Design review of the part built by this model. Coordinates are the model's own, in mm. A direction names the side the tool comes from. Coordinates: 2 decimals unless noted, no trailing zeros. Write each loop counter-clockwise with the first axis right and the second up, starting at its lowest first coordinate (ties: lowest second). Pieces come first, ordered by that corner, then holes. Notation, with made-up numbers: M 75,-33 L 131,-33 A16 ccw 131,-12 Z; hole C 9,87 d7. An arc over 180 degrees is marked long. Return JSON: item names as keys, results as strings. Group by question number.
```python
from build123d import *

# Parameters (mm, degrees)
CROQUIS1_W                = 110
CROQUIS1_H                = 60
SALIENTE_EXTRUIR1_DEPTH   = 5
SALIENTE_EXTRUIR2_DEPTH   = 45
CROQUIS4_W                = 15
CROQUIS4_H                = 15
SALIENTE_EXTRUIR3_DEPTH   = 15
CROQUIS5_W                = 15
CROQUIS5_H                = 15
CORTAR_EXTRUIR1_DEPTH     = 5
TALADRO_ROSCADO_M41_D     = 3.3
TALADRO_ROSCADO_M41_DEPTH = 14.008579979
TALADRO_ROSCADO_M41_TIP   = 0.991420021
CROQUIS11_W               = 5
CROQUIS11_H               = 4
SALIENTE_EXTRUIR4_DEPTH   = 3
CROQUIS12_W               = 40
CROQUIS12_H               = 4
SALIENTE_EXTRUIR5_DEPTH   = 2


with BuildPart() as part:
    # Croquis1 → Saliente-Extruir1 (new body)
    with BuildSketch(Plane(origin=(0, 0, 0), x_dir=(1, 0, 0), z_dir=(0, 1, 0))):
        with Locations((55, 30)):
            Rectangle(CROQUIS1_W, CROQUIS1_H)
    extrude(amount=SALIENTE_EXTRUIR1_DEPTH)

    # Croquis2 → Saliente-Extruir2 (add)
    with BuildSketch(Plane(origin=(0, 5, 0), x_dir=(1, 0, 0), z_dir=(0, 1, 0))):
        Polygon((0, 0), (10, 0), (10, 15), (5, 15), (5, 45), (10, 45), (10, 60), (0, 60), align=None)
    extrude(amount=SALIENTE_EXTRUIR2_DEPTH)

    # Croquis4 → Saliente-Extruir3 (add)
    with BuildSketch(Plane(origin=(0, 5, 0), x_dir=(1, 0, 0), z_dir=(0, 1, 0))):
        with Locations((102.5, 52.5)):
            Rectangle(CROQUIS4_W, CROQUIS4_H)
        with Locations((102.5, 7.5)):
            Rectangle(CROQUIS4_W, CROQUIS4_H)
    extrude(amount=SALIENTE_EXTRUIR3_DEPTH)

    # Croquis5 → Cortar-Extruir1 (cut)
    with BuildSketch(Plane(origin=(110, 0, 0), x_dir=(0, 0, -1), z_dir=(1, 0, 0))):
        with Locations((7.5, 12.5)):
            Rectangle(CROQUIS5_W, CROQUIS5_H)
        with Locations((52.5, 12.5)):
            Rectangle(CROQUIS5_W, CROQUIS5_H)
    extrude(amount=-CORTAR_EXTRUIR1_DEPTH, mode=Mode.SUBTRACT)

    # Taladro roscado M41
    with Locations(Plane(origin=(105, 0, 0), x_dir=(0, 0, -1), z_dir=(1, 0, 0))):
        with Locations((7.5, 12.5), (52.5, 12.5)):
            Hole(TALADRO_ROSCADO_M41_D / 2, depth=TALADRO_ROSCADO_M41_DEPTH)
            with Locations((0, 0, -(TALADRO_ROSCADO_M41_DEPTH + TALADRO_ROSCADO_M41_TIP / 2))):  # 118° drill point
                Cone(0, TALADRO_ROSCADO_M41_D / 2, TALADRO_ROSCADO_M41_TIP, mode=Mode.SUBTRACT)

    # Croquis11 → Saliente-Extruir4 (add)
    with BuildSketch(Plane.ZY):
        with Locations((-47.5, 32)):
            Rectangle(CROQUIS11_W, CROQUIS11_H)
        with Locations((-12.5, 32)):
            Rectangle(CROQUIS11_W, CROQUIS11_H)
    extrude(amount=SALIENTE_EXTRUIR4_DEPTH)

    # Croquis12 → Saliente-Extruir5 (add)
    with BuildSketch(Plane.ZY.offset(3)):
        with Locations((-30, 32)):
            Rectangle(CROQUIS12_W, CROQUIS12_H)
    extrude(amount=SALIENTE_EXTRUIR5_DEPTH)


solid = part.part
```
Item 1: Add section C-C (x = 7.5). Write out the cut boundary in (y, z), plus the area to 3 significant figures.
Item 2: The part is to be moulded in two halves that separate along X. For faces 4 (the flat face through (-1, 32, -45)), 5 (the flat face through (105, 14.3, -7.4)), 6 (the flat face through (54, 0, -30)), 7 (the flat face through (10, 27, -52)), say which applies: pulls with the +X half, pulls with the -X half, needs draft (parallel to the pull), parting line crosses it, or undercut.
Item 3: Machinability: for faces 1 (the flat face through (-2, 32, -10)), 2 (the flat face through (-3, 32, -30)), 3 (the flat face through (8, 27, -15)), which of the approach directions +Z, -Z, +X, -X, +Y, -Y give a long, thin tool a straight path to every point of the face, cutting with its end or side? Answer none if there is none.
Item 4: For line 1 (X direction, y = 17, z = -8); line 2 (Y direction, x = 98, z = -52.5); line 3 (Z direction, x = 102, y = 12), list the stretches that pass through material, from the lowest coordinate up.
Item 5: For pin 1 (1 mm diameter, centred on y = 22, z = -7.5, fed in from -X); pin 2 (3 mm diameter, centred on x = 98.5, z = -5, fed in from +Y); pin 3 (7.5 mm diameter, centred on y = 34, z = -51.5, fed in from +X), all flat-tipped, find the tip position at first contact; note any pin that passes through.
Item 6: Add section B-B (z = -7.5). Write out the cut boundary in (x, y), plus the area to 3 significant figures.
Item 7: Add section A-A (y = 12.5). Write out the cut boundary in (x, z), plus the area to 3 significant figures.
Item 8: Add section D-D (y = 32). Write out the cut boundary in (x, z).
Geometry check:
{
 "1": {"outline": "M 0,-60 L 50,-60 L 50,-45 L 5,-45 L 5,-15 L 50,-15 L 50,0 L 0,0 Z", "area": "1,650 mm^2"},
 "2": {"face 4": "undercut", "face 5": "pulls with the +X half", "face 6": "needs draft", "face 7": "undercut"},
 "3": {"face 1": "+Z, -X, +Y, -Y", "face 2": "+Y, -Y", "face 3": "+X, +Y"},
 "4": {"line 1": "0 to 10, 95 to 105", "line 2": "0 to 10.85, 14.15 to 20", "line 3": "-60 to -54.07, -50.93 to -45, -15 to -9.07, -5.93 to 0"},
 "5": {"pin 1": "x = 0", "pin 2": "y = 20", "pin 3": "x = 10"},
 "6": {"outline": "M 0,0 L 110,0 L 110,5 L 105,5 L 105,10.85 L 95,10.85 L 95,5 L 10,5 L 10,50 L 0,50 Z; M 95,14.15 L 105,14.15 L 105,20 L 95,20 Z", "area": "1,120 mm^2"},
 "7": {"outline": "M 0,-60 L 10,-60 L 10,-45 L 5,-45 L 5,-15 L 10,-15 L 10,0 L 0,0 Z; M 95,-60 L 105,-60 L 105,-54.15 L 95,-54.15 Z; M 95,-50.85 L 105,-50.85 L 105,-45 L 95,-45 Z; M 95,-15 L 105,-15 L 105,-9.15 L 95,-9.15 Z; M 95,-5.85 L 105,-5.85 L 105,0 L 95,0 Z", "area": "684 mm^2"},
 "8": {"outline": "M -5,-50 L 0,-50 L 0,-60 L 10,-60 L 10,-45 L 5,-45 L 5,-15 L 10,-15 L 10,0 L 0,0 L 0,-10 L -5,-10 Z; hole M -3,-45 L 0,-45 L 0,-15 L -3,-15 Z"}
}
